For this review, take the finished solid that the model builds, in its own axes (mm). A direction names the side the tool comes from. Give positions to 0.01 mm unless a question says otherwise; leave off trailing zeros. Loops run counter-clockwise (first coordinate to the right, second up) from the corner with the lowest first, then second, coordinate; pieces in that order, holes last.
```python
from build123d import *

# Parameters (mm, degrees)
F0_W     = 10
F0_H     = 30
F0_W_2   = 8
F0_H_2   = 15
F0_R     = 15.7140180489
F1_DEPTH = 15
F2_R     = 2


with BuildPart() as f1:
    # F0 (on Top) → F1 (new body)
    with BuildSketch(Plane.XY):
        Polygon((72.5661343038, 22.2410344053), (-82.4338656962, 22.2410344053), (-82.4338656962, -2.7589655947), (-72.4338656962, -2.7589655947), (-62.4338656962, -2.7589655947), (-54.4338656962, -2.7589655947), (-44.4338656962, -2.7589655947), (-30.4338656962, -2.7589655947), (72.5661343038, -2.7589655947), align=None)
        with Locations((-77.4338656962, -17.7589655947)):
            Rectangle(F0_W, F0_H)
        with Locations((-58.4338656962, -10.2589655947)):
            Rectangle(F0_W_2, F0_H_2)
        Polygon((-37.4338656962, -16.0254647561), (-30.4338656962, -2.7589655947), (-44.4338656962, -2.7589655947), align=None)
        with BuildLine():
            ThreePointArc((72.5661343038, -2.7589655947), (140.2578763804, 9.7410344053), (72.5661343038, 22.2410344053))
            Line((72.5661343038, 22.2410344053), (72.5661343038, -2.7589655947))
        make_face()
        with Locations((105.2578763804, 9.7410344053)):
            Circle(F0_R, mode=Mode.SUBTRACT)
    extrude(amount=F1_DEPTH)

    # F2
    f2_edges = [f1.edges().sort_by_distance(p)[0] for p in [
        (-82.433866, -5.258966, 15),
        (-4.933866, 22.241034, 15),
        (-72.433866, -17.758966, 15),
        (-77.433866, -32.758966, 15),
        (-67.433866, -2.758966, 15),
        (-62.433866, -10.258966, 15),
        (-58.433866, -17.758966, 15),
        (-54.433866, -10.258966, 15),
        (-40.933866, -9.392215, 15),
        (21.066134, -2.758966, 15),
        (-33.933866, -9.392215, 15),
        (140.257876, 9.741034, 15),
        (-49.433866, -2.758966, 15),
    ]]
    fillet(f2_edges, radius=F2_R)


solid = f1.part
```
Q1. Consider section A-A on z = 9. Give the boundary of the cut face in (x, y), plus the area to 3 significant figures.
Answers:
outline: (-82.43, -32.76) - (-72.43, -32.76) - (-72.43, -2.76) - (-62.43, -2.76) - (-62.43, -17.76) - (-54.43, -17.76) - (-54.43, -2.76) - (-44.43, -2.76) - (-37.43, -16.03) - (-30.43, -2.76) - (72.57, -2.76) arc R35 ccw (long way) to (72.57, 22.24) - (-82.43, 22.24) - close; hole circle Ø31.43 at (105.26, 9.74)
area: 7,420 mm2
Q2. Mouldability with a two-part tool opening along Y and no side actions: class faces 4 (the flat face through (52, 7, 0)), 5 (the cylindrical face through (119.774, 3.722, 7.395)), 6 (the flat face through (-50, -2.759, 6)) as +Y half, -Y half, draft (parallel to the pull), parting line (faces both ways), or undercut.
Answers:
face 4: draft
face 5: undercut
face 6: -Y half
Q3. Consider section B-B on x = 55. Give the boundary of the cut face in (y, z), plus the area to 3 significant figures.
Answers:
outline: (-2.76, 0) - (22.24, 0) - (22.24, 13) arc R2 ccw to (20.24, 15) - (-0.76, 15) arc R2 ccw to (-2.76, 13) - close
area: 373 mm2
Q4. For pin 1 Ø8 at (x, y) = (23, -8.5) entering from +Z; pin 2 Ø6 at (y, z) = (-21.5, 3) entering from +X; pin 3 Ø4 at (x, z) = (-22.5, 8.5) entering from +Y; pin 4 Ø8 at (x, z) = (-69, 7) entering from -Y, all flat-tipped, find the tip position at first contact; note any pin that passes through.
Answers:
pin 1: passes through
pin 2: stops at x = 125.93
pin 3: stops at y = 22.24
pin 4: stops at y = -32.76
Q5. Machinability: for faces 1 (the cylindrical face through (-34.104, -8.492, 14.399)), 2 (the flat face through (-4, 22.241, 6)), 3 (the flat face through (-62.434, -10, 6)), which of the approach directions +Z, -Z, +X, -X, +Y, -Y give a long, thin tool a straight path to every point of the face, cutting with its end or side? Answer none if there is none.
Answers:
face 1: +Z, -Y
face 2: +Z, -Z, -X, +Y
face 3: +Z, -Z, -Y
Q6. For probe 1 along X at (y, z) = (-16.5, 12.25); probe 2 along X at (y, z) = (-7.5, 12); probe 3 along X at (y, z) = (-8, 8.5), list the stretches that pass through material, from the lowest coordinate up.
Answers:
probe 1: x = -82.43 to -72.43, -62.43 to -54.43, 82.1 to 128.42
probe 2: x = -82.43 to -72.43, -62.43 to -54.43, -41.93 to -32.94, 74.8 to 135.72
probe 3: x = -82.43 to -72.43, -62.43 to -54.43, -41.67 to -33.2, 75.09 to 135.43
